Autodesk Inventor part; units mm, degrees
ref_plane "Work Plane3" through (0, 0, 0) normal (0, 1, 0) x (-1, 0, 0)
ref_plane "YZ Plane" through (0, 0, 0) normal (1, 0, 0) x (0, 1, 0)
ref_plane "XY Plane" through (0, 0, 0) normal (0, 0, 1) x (1, 0, 0)
sketch "Sketch1" plane through (0, 0, 0) normal (0, 0, 1) x (1, 0, 0)
  arc A0 (9.7855, 7.7778) -> (9.7855, -7.7778) centre (0, 0) ccw
  circle A1 centre (0, 0) radius 11
  arc A2 (60, -4) -> (60, 4) centre (60, 0) ccw
  line L0 (60, 4) -> (17.6139, 4) construction
  line L1 (60, -4) -> (17.6139, -4) construction
  arc A3 (17.6139, -4) -> (9.7855, -7.7778) centre (17.6139, -14) ccw
  arc A4 (9.7855, 7.7778) -> (17.6139, 4) centre (17.6139, 14) ccw
  line L2 (30, 4) -> (30, -4) construction
  line L3 (17.6139, -4) -> (17.6139, 4)
  point P0 (11.8427, 4)
  point P1 (11.8427, -4)
  point P2 (-12.5, 0)
  point P3 (30, 0)
  dimension "d0" = 25
  dimension "d1" = 22
  dimension "d2" = 4
  dimension "d3" = 10
  dimension "d4" = 60
  dimension "d17" = 42.5
extrude "Extrusion1" add sketch "Sketch1" against normal blind 3
ref_plane "Work Plane3" through (0, 0, 0) normal (0, 1, 0) x (-1, 0, 0)
sketch "Sketch7" plane through (0, 0, 0) normal (0, 1, 0) x (-1, 0, 0)
  line L0 (-17.6139, 0) -> (-17.6139, -3)
  line L1 (-17.6139, -3) -> (-30, -3)
  line L2 (-30, -3) -> (-46, -4.5)
  line L3 (-46, -4.5) -> (-60, -4.5)
  line L4 (-60, -4.5) -> (-60, -1.5)
  line L5 (-60, -1.5) -> (-46, -1.5)
  line L6 (-46, -1.5) -> (-30, 0)
  line L7 (-30, 0) -> (-17.6139, 0)
  line L8 (-17.6139, -3) -> (-17.6139, 0)
  point P0 (0, 0)
  point P1 (-60, -3)
  dimension "d19" = 1.5
  dimension "d20" = 14
  dimension "d21" = 60
  dimension "d22" = 3
extrude "Extrusion3" add sketch "Sketch7" along normal mid plane 8
sketch "Sketch8" plane through (46, 4, -1.5) normal (0, 0, 1) x (1, 0, 0)
  line L0 (14, -8) -> (14, 0)
  arc A0 (14, -8) -> (14, 0) centre (14, -4) ccw
  point P0 (-46, -4)
  dimension "d25" = 4
extrude "Extrusion4" add sketch "Sketch8" against normal up to surface (3 mm away)
sketch "Sketch9" plane through (46, -4, -1.5) normal (0, 0, 1) x (1, 0, 0)
  arc A0 (14, 0) -> (14, 8) centre (14, 4) ccw
  point P0 (-46, 4)
hole "Hole1" at (60, 0, -1.5) direction (0, 0, -1) diameter 5 depth 3
properties part number "15B"
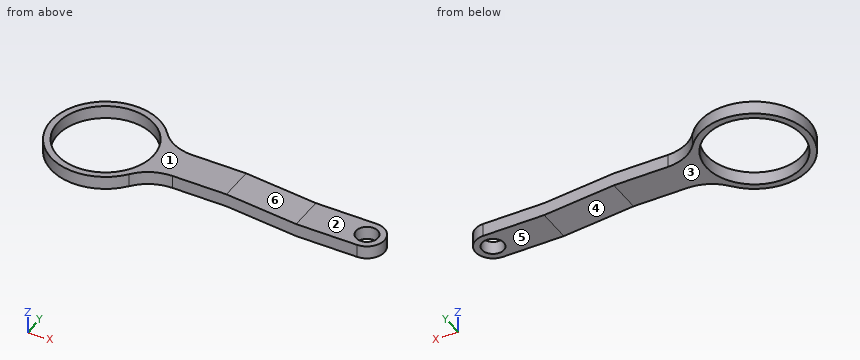
Source: CAD feature listing. Evaluate the final solid. Frame: model axes, mm. Face numbers are marked on the shaded views. A direction names the side the tool comes from. Round coordinates to 2 decimals unless told otherwise and drop trailing zeros. Loops run counter-clockwise (first coordinate to the right, second up) from the corner with the lowest first, then second, coordinate; pieces in that order, holes last.
Q1. Ray query, line 1 (Y direction, x = 0, z = -2.4); line 2 (Y direction, x = 60, z = -2.45); line 3 (X direction, y = -1.5, z = -2.95). Return the intervals inside material, ascending.
Q2. Access query for the marked faces 1, 2 and 3. Directions: +Z, -Z, +X, -X, +Y, -Y. A direction counts if a zero-diameter tool reaches every point of the face in a straight line with its end or side. Return the directions, or none.
Q3. Section D-D, the plane x = 43. Return loops of the section in (y, z).
Q4. Mould query, pull axis X, two halves, no side actions, for the marked faces 4, 5 and 6. Classes: pulls with the +X half, pulls with the -X half, needs draft (parallel to the pull), parting line crosses it, or undercut.
Q5. Section A-A, the plane y = 0. Return loops of the section in (x, z), plus the area to 4 significant figures.
Q6. Section B-B, the plane x = 0. Return loops of the section in (y, z), plus the area to 3 significant figures.
Q7. Section C-C, the plane y = -9.5. Return loops of the section in (x, z), plus the area to 3 significant figures.
Q8. First-contact query: P1, Ø2, axis at y = -9, z = -1.5, coming from the +X side; P2, Ø12, axis at x = 34.5, y = 4.5, coming from the -Z side; P3, Ø12.5, axis at x = 12, y = 0.5, coming from the -Z side. Flat tips, straight axial feed; report the tip coordinate or a pass-through.
Solutions:
1. line 1: y = -12.5 to -11, 11 to 12.5
1. line 2: y = -4 to -2.5, 2.5 to 4
1. line 3: x = -12.41 to -10.9, 10.9 to 58, 62 to 63.71
2. face 1: +Z, +X, -X, +Y, -Y
2. face 2: +Z, +X, +Y, -Y
2. face 3: -Z, -X, +Y, -Y
3. outline: (-4, -4.22) - (4, -4.22) - (4, -1.22) - (-4, -1.22) - close
4. face 4: pulls with the -X half
4. face 5: needs draft
4. face 6: pulls with the +X half
5. outline: (-12.5, -3) - (-11, -3) - (-11, 0) - (-12.5, 0) - close; (11, -3) - (30, -3) - (46, -4.5) - (57.5, -4.5) - (57.5, -1.5) - (46, -1.5) - (30, 0) - (11, 0) - close; (62.5, -4.5) - (64, -4.5) - (64, -1.5) - (62.5, -1.5) - close
5. area: 148.5 mm2
6. outline: (-12.5, -3) - (-11, -3) - (-11, 0) - (-12.5, 0) - close; (11, -3) - (12.5, -3) - (12.5, 0) - (11, 0) - close
6. area: 9.00 mm2
7. outline: (-8.12, -3) - (-5.55, -3) - (-5.55, 0) - (-8.12, 0) - close; (5.55, -3) - (8.12, -3) - (8.12, 0) - (5.55, 0) - close
7. area: 15.5 mm2
8. P1: stops at x = 9.6
8. P2: stops at z = -3.98
8. P3: stops at z = -3
